Could you check a few things on this drawing? It's one solid part, dimensions in mm from its lowest x, y, z. A direction names the side the tool comes from. Coordinates: 2 decimals unless noted, no trailing zeros. Write each loop counter-clockwise with the first axis right and the second up, starting at its lowest first coordinate (ties: lowest second). Pieces come first, ordered by that corner, then holes. Notation, with made-up numbers: M 48.25,-2 L 72.25,-2 A23 ccw 72.25,24 Z; hole C -10,-33.5 d6. An arc over 180 degrees is marked long. Use a Markdown table: item, result.
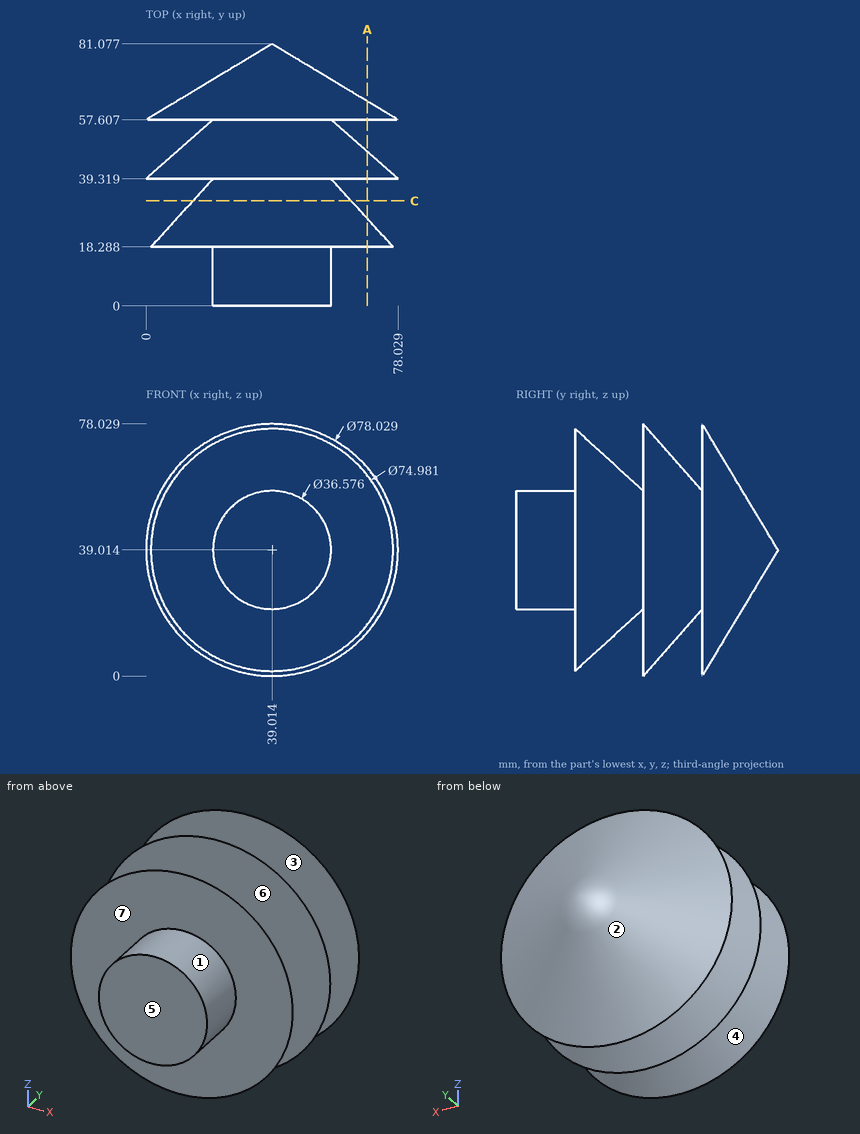
1. We'd pull the mould along Y, two halves only. Please class the marked faces 1, 2, 3 and 4: +Y half, -Y half, draft (parallel to the pull), parting line (faces both ways), or undercut.
Answers follow:
| item | result |
|---|---|
| face 1 | draft |
| face 2 | +Y half |
| face 3 | undercut |
| face 4 | undercut |
2. Which directions (+Z, -Z, +X, -X, +Y, -Y) give clear straight access to the entire face, cutting with the end or side of a thin tool? Please do the marked faces 5, 6 and 7.
Answers follow:
| item | result |
|---|---|
| face 5 | +Z, -Z, +X, -X, -Y |
| face 6 | none |
| face 7 | -Y |
3. Suppose I cut it at A-A on x = 68.5. State how many separate pieces and enclosed holes the cut face has, and give its area (3 significant figures).
Answers follow:
| item | result |
|---|---|
| separate pieces | 3 |
| enclosed holes | 0 |
| area | 732 mm2 |
4. Will these pins go through, and if not, where does the flat tip stop? pin 1 Ø6 at (x, z) = (41.5, 15.5) entering from -Y; pin 2 Ø1.5 at (x, z) = (24.5, 55) entering from +Y; pin 3 Ø2 at (y, z) = (38, 15.5) entering from +X; pin 4 Ø10 at (x, z) = (8, 57) entering from +Y.
Answers follow:
| item | result |
|---|---|
| pin 1 | stops at y = 18.29 |
| pin 2 | stops at y = 68.54 |
| pin 3 | passes through |
| pin 4 | stops at y = 62.52 |
5. I need wall thicknesses on probe 1 along Y at (x, z) = (63, 32) (1 decimal); probe 2 along Y at (x, z) = (64.5, 40.5) (1 decimal); probe 3 along Z at (x, y) = (63.5, 23) (1 decimal). Which ranges of each line are inside material? Lowest first, please.
Answers follow:
| item | result |
|---|---|
| probe 1 | y = 18.3 to 32, 39.3 to 51.7, 57.6 to 66 |
| probe 2 | y = 18.3 to 31.4, 39.3 to 51.2, 57.6 to 65.7 |
| probe 3 | z = 16.6 to 61.4 |
6. Suppose I cut it at C-C on y = 32.5. Write out the boundary of the cut face in (x, z) (1 decimal), and give its area (3 significant figures).
Answers follow:
| item | result |
|---|---|
| outline | C 39,39 d49 |
| area | 1,890 mm2 |
